Source: CAD feature listing. Evaluate the final solid. Frame: model axes, mm. Give positions to 0.01 mm unless a question says otherwise; leave off trailing zeros. Loops run counter-clockwise (first coordinate to the right, second up) from the corner with the lowest first, then second, coordinate; pieces in that order, holes last. Notation, with made-up numbers: (82, 12) - (129, 12) arc R12 cw to (129, 18) - close; hole circle Ø4 at (17.5, 30.25). An arc over 180 degrees is marked (long way). Put each result on its own line as item: value.
```python
from build123d import *

# Parameters (mm, degrees)
F2_T      = -3
F4_D      = 3
F4_DEPTH  = 10.501
F6_D      = 3
F8_D      = 3
F8_DEPTH  = 10.501
F10_D     = 3
F12_D     = 3
F12_DEPTH = 10.501
F14_D     = 3


with BuildPart() as f1:
    # F0 (on Top) → F1 (revolve)
    with BuildSketch(Plane.XY):
        with BuildLine():
            ThreePointArc((10.5, 0), (0, 10.5), (-10.5, 0))
            Line((-10.5, 0), (10.5, 0))
        make_face()
    revolve(axis=Axis((0.3997717993, 0, 0), (1, 0, 0)))

    # F2 (hollow: no face is removed)
    offset(amount=F2_T, mode=Mode.SUBTRACT)

    # F4 (through all, one way)
    with BuildSketch(Plane.XY):
        with Locations((0, 0)):
            Circle(F4_D / 2)
    extrude(amount=-F4_DEPTH, mode=Mode.SUBTRACT)

    # F6 (through all)
    with Locations(Plane(origin=(0, 0, 0), x_dir=(1, 0, 0), z_dir=(0, 0, -1))):
        with Locations((0, 0)):
            Hole(F6_D / 2)

    # F8 (through all, one way)
    with BuildSketch(Plane.YZ):
        with Locations((0, 0)):
            Circle(F8_D / 2)
    extrude(amount=-F8_DEPTH, mode=Mode.SUBTRACT)

    # F10 (through all)
    with Locations(Plane(origin=(0, 0, 0), x_dir=(0, 1, 0), z_dir=(-1, 0, 0))):
        with Locations((0, 0)):
            Hole(F10_D / 2)

    # F12 (through all, one way)
    with BuildSketch(Plane.XZ):
        with Locations((0, 0)):
            Circle(F12_D / 2)
    extrude(amount=-F12_DEPTH, mode=Mode.SUBTRACT)

    # F14 (through all)
    with Locations(Plane(origin=(0, 0, 0), x_dir=(1, 0, 0), z_dir=(0, 1, 0))):
        with Locations((0, 0)):
            Hole(F14_D / 2)


solid = f1.part
```
1) Section query A-A, the plane x = 0. Output: boundary loops of the cut face in (y, z).
Check result:
outline: (-10.39, -1.5) arc R10.5 ccw to (-1.5, -10.39) - (-1.5, -7.35) arc R7.5 cw to (-7.35, -1.5) - close; (-10.39, 1.5) - (-7.35, 1.5) arc R7.5 cw to (-1.5, 7.35) - (-1.5, 10.39) arc R10.5 ccw to start; (1.5, -10.39) arc R10.5 ccw to (10.39, -1.5) - (7.35, -1.5) arc R7.5 cw to (1.5, -7.35) - close; (1.5, 7.35) arc R7.5 cw to (7.35, 1.5) - (10.39, 1.5) arc R10.5 ccw to (1.5, 10.39) - close
2) Mould query, pull axis Z, two halves, no side actions, for faces 1 (the cylindrical face through (-1.5, 0.07, -8.85)), 2 (the cylindrical face through (1.5, -8.89, -0.07)). Classes: pulls with the +Z half, pulls with the -Z half, needs draft (parallel to the pull), parting line crosses it, or undercut.
Check result:
face 1: needs draft
face 2: undercut
3) Material intervals for line 1 along Z through (x, y) = (-0.75, -5.5); line 2 along Z through (x, y) = (1, 5.25); line 3 along Y through (x, z) = (0, 7.5), sorted ascending. Write a range as [from, to].
Check result:
line 1: [-8.91, -5.04], [5.04, 8.91]
line 2: [-9.04, -5.26], [5.26, 9.04]
line 3: [-7.35, -1.5], [1.5, 7.35]
4) Section query D-D, the plane x = 9.25. Output: boundary loops of the cut face in (y, z).
Check result:
outline: circle Ø9.94 at (0, 0); hole circle Ø3 at (0, 0)
5) Section query C-C, the plane z = 4. Output: boundary loops of the cut face in (x, y).
Check result:
outline: circle Ø19.42 at (0, 0); hole circle Ø12.69 at (0, 0)
6) Pin query (flat end, axial travel): P1, Ø1, axis at x = 3, y = -7.5, coming from the -Z side; P2, Ø1, axis at x = -4, y = -5.5, coming from the -Z side; P3, Ø2.5, axis at x = 0, z = 0, coming from the -Y side; P4, Ø6, axis at x = 5, y = -4, coming from the +Z side. Return the tip coordinate at first contact, or that it passes through.
Check result:
P1: z = -7.27
P2: z = -8.4
P3: through
P4: z = 9.93
